For this review, take the finished solid that the model builds, in its own axes (mm). A direction names the side the tool comes from. Give positions to 0.01 mm unless a question says otherwise; leave off trailing zeros. Order: outer loops, then holes, each group sorted by start corner. A loop starts at its lowest first (then second) coordinate and runs counter-clockwise, first axis right, second up. Notation, with made-up numbers: (-7, 39.25) -> (7, 39.25) arc R14 ccw to (7, 56.25) -> close; hole circle Ø10 at (-39.5, 59.25). An arc over 180 degrees is marked (long way). Return JSON: item names as keys, results as strings. Group by question number.
1) Add section C-C (z = -10). Give the boundary of the cut face in (x, y), then the cut area to 3 significant figures.
2) The part is to be moulded in two halves that separate along X. For faces 1 (the face through (0, 10, -15)), 2 (the face through (-0.54, 12.56, 9.93)), 3 (the face through (-0.54, 12.56, -9.93)), 4 (the face through (10, -2, 0)), say which applies: released by +X, released by -X, zero draft, split by the parting line, or undercut.
3) Add section D-D (x = -6.5). Give the boundary of the cut face in (y, z), then the cut area to 3 significant figures.
4) Add section A-A (x = 0). Give the boundary of the cut face in (y, z), then the cut area to 3 significant figures.
5) To check wall thickness, follow line 1 along Y through (x, z) = (0, 7.75); line 2 along Z through (x, y) = (-2, 23); line 3 along Y through (x, z) = (-4.75, -1). State the ranges of each line that lie inside material, in increasing order.
6) For faces 5 (the face through (0, 10, 5)), 6 (the face through (0, 25, -10)), list the 3-axis set-ups (+Z, -Z, +X, -X, +Y, -Y) from which the entire face can be reached by the end or side of a thin tool; tool diameter is ignored.
7) Add section B-B (y = 3). Give the boundary of the cut face in (x, z), then the cut area to 3 significant figures.
8) Insertion check: P1, Ø3, axis at x = 0, y = 15, coming from the -Z side; P2, Ø6, axis at x = 4, z = -11.5, coming from the +Y side; P3, Ø1.5, axis at x = -5, z = -7.5, coming from the +Y side. Each pin has a flat end and moves straight along its axis. Give the tip position at first contact, or say it passes through.
from build123d import *

# Parameters (mm, degrees)
BOSS_EXTRUDE1_START = 5
SKETCH1_R           = 2.5
BOSS_EXTRUDE1_DEPTH = 10
BOSS_EXTRUDE2_START = -5
SKETCH1_2_R         = 2.5
BOSS_EXTRUDE2_DEPTH = 10
SKETCH2_W           = 20
SKETCH2_H           = 30
BOSS_EXTRUDE3_DEPTH = 5


with BuildPart() as part:
    # Sketch1 → Boss-Extrude1 (new body)
    with BuildSketch(Plane.XY.offset(BOSS_EXTRUDE1_START)):
        with BuildLine():
            Line((-10, 15), (-10, 0))
            Line((-10, 0), (10, 0))
            Line((10, 0), (10, 15))
            ThreePointArc((10, 15), (0, 25), (-10, 15))
        make_face()
        with Locations((0, 15)):
            Circle(SKETCH1_R, mode=Mode.SUBTRACT)
    extrude(amount=BOSS_EXTRUDE1_DEPTH)



with BuildPart() as body_2:
    # Sketch1<2> → Boss-Extrude2 (new body)
    with BuildSketch(Plane.XY.offset(BOSS_EXTRUDE2_START)):
        with BuildLine():
            Line((-10, 15), (-10, 0))
            Line((-10, 0), (10, 0))
            Line((10, 0), (10, 15))
            ThreePointArc((10, 15), (0, 25), (-10, 15))
        make_face()
        with Locations((0, 15)):
            Circle(SKETCH1_2_R, mode=Mode.SUBTRACT)
    extrude(amount=-BOSS_EXTRUDE2_DEPTH)


with BuildPart() as part_1:
    add(part.part)

    add(body_2.part)  # Boss-Extrude3 merges body 2
    # Sketch2 → Boss-Extrude3 (add)
    with BuildSketch(Plane.XZ):
        Rectangle(SKETCH2_W, SKETCH2_H)
    extrude(amount=BOSS_EXTRUDE3_DEPTH)


solid = part_1.part
Evaluation:
{
 "1": {"outline": "(-10, -5) -> (10, -5) -> (10, 15) arc R10 ccw to (-10, 15) -> close; hole circle Ø5 at (0, 15)", "area": "537 mm^2"},
 "2": {"face 1": "zero draft", "face 2": "undercut", "face 3": "undercut", "face 4": "released by +X"},
 "3": {"outline": "(-5, -15) -> (22.6, -15) -> (22.6, -5) -> (0, -5) -> (0, 5) -> (22.6, 5) -> (22.6, 15) -> (-5, 15) -> close", "area": "602 mm^2"},
 "4": {"outline": "(-5, -15) -> (12.5, -15) -> (12.5, -5) -> (0, -5) -> (0, 5) -> (12.5, 5) -> (12.5, 15) -> (-5, 15) -> close; (17.5, -15) -> (25, -15) -> (25, -5) -> (17.5, -5) -> close; (17.5, 5) -> (25, 5) -> (25, 15) -> (17.5, 15) -> close", "area": "550 mm^2"},
 "5": {"line 1": "-5 to 12.5, 17.5 to 25", "line 2": "-15 to -5, 5 to 15", "line 3": "-5 to 0"},
 "6": {"face 5": "+X, -X, +Y", "face 6": "+Z, -Z, +Y"},
 "7": {"outline": "(-10, -15) -> (10, -15) -> (10, -5) -> (-10, -5) -> close; (-10, 5) -> (10, 5) -> (10, 15) -> (-10, 15) -> close", "area": "400 mm^2"},
 "8": {"P1": "through", "P2": "y = 24.95", "P3": "y = 24.05"}
}
